```python
from build123d import *

# Parameters (mm, degrees)
SKETCH1_W           = 13.97
SKETCH1_H           = 19.05
SKETCH1_R           = 1.5875
BOSS_EXTRUDE1_DEPTH = 1.27
SKETCH2_R           = 4.5212
BOSS_EXTRUDE2_DEPTH = 17.0434
SKETCH3_W           = 2.413
SKETCH3_H           = 2.413
BOSS_EXTRUDE3_DEPTH = 2.413
SKETCH4_W           = 0.635
SKETCH4_H           = 0.635
BOSS_EXTRUDE4_DEPTH = 5.715


with BuildPart() as part:
    # Sketch1 → Boss-Extrude1 (new body)
    with BuildSketch(Plane.XY):
        with Locations((6.985, 9.525)):
            Rectangle(SKETCH1_W, SKETCH1_H)
        with Locations((2.54, 16.51)):
            Circle(SKETCH1_R, mode=Mode.SUBTRACT)
        with Locations((11.43, 2.54)):
            Circle(SKETCH1_R, mode=Mode.SUBTRACT)
    extrude(amount=BOSS_EXTRUDE1_DEPTH)

    # Sketch2 → Boss-Extrude2 (add)
    with BuildSketch(Plane.XY.offset(1.27)):
        with Locations((5.08, 6.35)):
            Circle(SKETCH2_R)
    extrude(amount=BOSS_EXTRUDE2_DEPTH)

    # Sketch3 → Boss-Extrude3 (add)
    with BuildSketch(Plane(origin=(0, 0, 0), x_dir=(-1, 0, 0), z_dir=(0, 0, -1))):
        with Locations((-14.4145, 9.8425)):
            Rectangle(SKETCH3_W, SKETCH3_H)
        with Locations((-14.4145, 12.3825)):
            Rectangle(SKETCH3_W, SKETCH3_H)
        with Locations((-14.4145, 14.9225)):
            Rectangle(SKETCH3_W, SKETCH3_H)
        with Locations((-14.4145, 17.4625)):
            Rectangle(SKETCH3_W, SKETCH3_H)
    extrude(amount=BOSS_EXTRUDE3_DEPTH)

    # Sketch4 → Boss-Extrude4 (add)
    with BuildSketch(Plane(origin=(15.621, 0, 0), x_dir=(0, 0, -1), z_dir=(1, 0, 0))):
        with Locations((1.2065, 9.8425)):
            Rectangle(SKETCH4_W, SKETCH4_H)
        with Locations((1.2065, 12.3825)):
            Rectangle(SKETCH4_W, SKETCH4_H)
        with Locations((1.2065, 14.9225)):
            Rectangle(SKETCH4_W, SKETCH4_H)
        with Locations((1.2065, 17.4625)):
            Rectangle(SKETCH4_W, SKETCH4_H)
    extrude(amount=BOSS_EXTRUDE4_DEPTH)


solid = part.part
```
Geometry check sheet. Reference: the model listing, model coordinates, mm. A direction names the side the tool comes from. Coordinates: 2 decimals unless noted, no trailing zeros. Loops run counter-clockwise (first coordinate to the right, second up) from the corner with the lowest first, then second, coordinate; pieces in that order, holes last. Notation, with made-up numbers: (35.5, 84.25) -> (94.5, 84.25) arc R24 ccw to (94.5, 115.25) -> close; hole circle Ø11 at (-22.5, 43.25). An arc over 180 degrees is marked (long way). Put each result on its own line as item: value.
1) Cross-section at B-B on x = 19.5. Record the boundary of the cut face in (y, z) (3 decimals).
Result set:
outline: (9.525, -1.524) -> (10.16, -1.524) -> (10.16, -0.889) -> (9.525, -0.889) -> close; (12.065, -1.524) -> (12.7, -1.524) -> (12.7, -0.889) -> (12.065, -0.889) -> close; (14.605, -1.524) -> (15.24, -1.524) -> (15.24, -0.889) -> (14.605, -0.889) -> close; (17.145, -1.524) -> (17.78, -1.524) -> (17.78, -0.889) -> (17.145, -0.889) -> close
2) Tool access check on faces 4 (the flat face through (14, 12, -2.413)), 5 (the flat face through (0, 9, 1)), 6 (the flat face through (15, 17, 0)), 7 (the flat face through (13.208, 17, -1)), 8 (the flat face through (14, 18.669, -1)). Record the directions out of +Z, -Z, +X, -X, +Y, -Y that give a thin tool (end or side, any length) a straight path to the whole face; none if there is none.
Result set:
face 4: -Z, +X, -X, +Y, -Y
face 5: +Z, -Z, -X, +Y, -Y
face 6: +Z, +X, +Y, -Y
face 7: -Z, -X, +Y, -Y
face 8: -Z, +X, -X, +Y
3) Cross-section at D-D on y = 6.35. Record the boundary of the cut face in (x, z).
Result set:
outline: (0, 0) -> (13.97, 0) -> (13.97, 1.27) -> (9.6, 1.27) -> (9.6, 18.31) -> (0.56, 18.31) -> (0.56, 1.27) -> (0, 1.27) -> close
4) Thickness scan on line 1 (Y direction, x = 2.54, z = 1); line 2 (Z direction, x = 12.25, y = 11.5); line 3 (Z direction, x = 7, y = 4.5). Record the ranges inside material, lowest first.
Result set:
line 1: y = 0 to 14.92, 18.1 to 19.05
line 2: z = 0 to 1.27
line 3: z = 0 to 18.31
5) Release check for a two-part mould opening along X. For faces 1 (the flat face through (13.208, 10, -1)), 2 (the flat face through (5, 6, 18.313)), 3 (the cylindrical face through (12.896, 1.932, 0.626)) record: released by +X, released by -X, zero draft, split by the parting line, or undercut.
Result set:
face 1: released by -X
face 2: zero draft
face 3: undercut
6) Gauge pin test, flat ends, axial feed: pin 1 Ø8 at (y, z) = (17, 9) entering from +X (3 decimals); pin 2 Ø1.2 at (y, z) = (15.5, -1) entering from -X; pin 3 Ø0.5 at (x, y) = (15, 17) entering from +Z; pin 4 Ø4 at (x, y) = (9.5, 10) entering from -Z. Record the tip position at first contact, or that the pin passes through.
Result set:
pin 1: passes through
pin 2: stops at x = 13.21
pin 3: stops at z = 0
pin 4: stops at z = 0
7) Cross-section at C-C on z = -0.5. Record the boundary of the cut face in (x, y).
Result set:
outline: (13.21, 8.64) -> (15.62, 8.64) -> (15.62, 11.05) -> (13.21, 11.05) -> close; (13.21, 11.18) -> (15.62, 11.18) -> (15.62, 13.59) -> (13.21, 13.59) -> close; (13.21, 13.72) -> (15.62, 13.72) -> (15.62, 16.13) -> (13.21, 16.13) -> close; (13.21, 16.26) -> (15.62, 16.26) -> (15.62, 18.67) -> (13.21, 18.67) -> close
8) Cross-section at A-A on x = 11.43. Record the boundary of the cut face in (y, z), plus the area to 3 significant figures.
Result set:
outline: (0, 0) -> (0.95, 0) -> (0.95, 1.27) -> (0, 1.27) -> close; (4.13, 0) -> (19.05, 0) -> (19.05, 1.27) -> (4.13, 1.27) -> close
area: 20.2 mm^2
